Source: CAD feature listing. Evaluate the final solid. Frame: model axes, mm. Face numbers are marked on the shaded views. A direction names the side the tool comes from. Round coordinates to 2 decimals unless told otherwise and drop trailing zeros. Write each loop counter-clockwise with the first axis right and the second up, starting at its lowest first coordinate (ties: lowest second). Pieces come first, ordered by that corner, then holes. Notation, with made-up numbers: M 70,53.25 L 114,53.25 A32 cw 114,79.25 Z; hole C -18,21.25 d5. An arc over 180 degrees is marked long. Answer in a Markdown table with one row per item. Add a question column.
Item 1: Cut plane A-A on x = -10.5. Return loops of the section in (y, z).
Item 2: Cut plane C-C on y = -5.5. Return loops of the section in (x, z).
Item 3: Contact query for flat-ended pins moving along their axis: pin 1 (2 mm diameter, centred on x = -15.5, z = 7, fed in from -Y); pin 2 (3 mm diameter, centred on y = 19, z = 1.5, fed in from -X); pin 3 (5 mm diameter, centred on x = -2.5, z = 8, fed in from -Y). Output: stop coordinate, or through.
Item 4: Material intervals for probe 1 along Z at (x, y) = (-9.75, -3); probe 2 along X at (y, z) = (3, 9.75); probe 3 along Y at (x, z) = (-12.5, 6.25), sorted ascending.
Item 5: Set-up query: the marked faces 4, 5 and 6. Return all of +Z, -Z, +X, -X, +Y, -Y with unobstructed straight access to the full face (end or side cutting, diameter ignored); none if empty.
Item 6: Mould query, pull axis Z, two halves, no side actions, for the marked faces 1, 2 and 3. Classes: released by +Z, released by -Z, zero draft, split by the parting line, or undercut.
Item 7: Cut plane D-D on z = 5. Return loops of the section in (x, y).
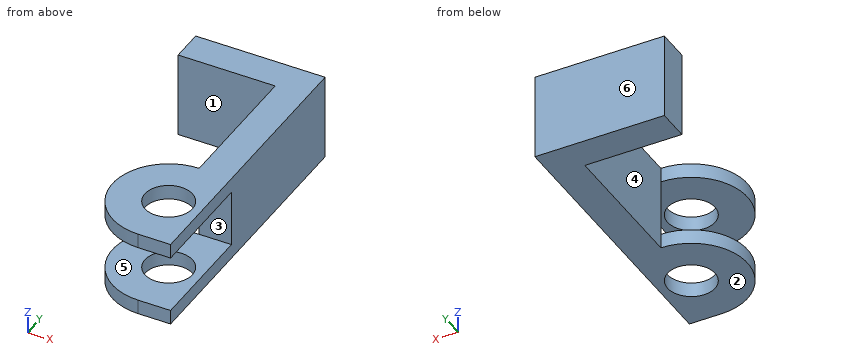
from build123d import *

# Parameters (mm, degrees)
SKETCH1_R           = 3.4925
BOSS_EXTRUDE1_DEPTH = 12.7
SKETCH2_W           = 25.4
SKETCH2_H           = 8.382
CUT_EXTRUDE1_DEPTH  = 16.51


with BuildPart() as part:
    # Sketch1 → Boss-Extrude1 (new body)
    with BuildSketch(Plane.XY):
        with BuildLine():
            Line((0, 0), (0, 25.4))
            Line((0, 25.4), (-19.05, 25.4))
            Line((-19.05, 25.4), (-19.05, 20.6375))
            Line((-19.05, 20.6375), (-4.7625, 20.6375))
            Line((-4.7625, 20.6375), (-4.7625, 0))
            ThreePointArc((-4.7625, 0), (-13.0175, -8.255), (-4.7625, -16.51))
            Line((-4.7625, -16.51), (0, -16.51))
            Line((0, -16.51), (0, 0))
        make_face()
        with Locations((-4.7625, -8.255)):
            Circle(SKETCH1_R, mode=Mode.SUBTRACT)
    extrude(amount=BOSS_EXTRUDE1_DEPTH)

    # Sketch2 → Cut-Extrude1 (cut)
    with BuildSketch(Plane.XZ.offset(16.51)):
        with Locations((-12.7, 6.35)):
            Rectangle(SKETCH2_W, SKETCH2_H)
    extrude(amount=-CUT_EXTRUDE1_DEPTH, mode=Mode.SUBTRACT)


solid = part.part
Results below:
| question | item | result |
|---|---|---|
| 1 | outline | M -14.19,0 L -2.32,0 L -2.32,2.16 L -14.19,2.16 Z; M -14.19,10.54 L -2.32,10.54 L -2.32,12.7 L -14.19,12.7 Z; M 20.64,0 L 25.4,0 L 25.4,12.7 L 20.64,12.7 Z |
| 2 | outline | M -12.54,0 L -6.91,0 L -6.91,2.16 L -12.54,2.16 Z; M -12.54,10.54 L -6.91,10.54 L -6.91,12.7 L -12.54,12.7 Z; M -2.62,0 L 0,0 L 0,2.16 L -2.62,2.16 Z; M -2.62,10.54 L 0,10.54 L 0,12.7 L -2.62,12.7 Z |
| 3 | pin 1 | y = 20.64 |
| 3 | pin 2 | x = -4.76 |
| 3 | pin 3 | y = 0 |
| 4 | probe 1 | 0 to 2.16, 10.54 to 12.7 |
| 4 | probe 2 | -4.76 to 0 |
| 4 | probe 3 | 20.64 to 25.4 |
| 5 | face 4 | +Z, -Z, -X |
| 5 | face 5 | +X, -X, -Y |
| 5 | face 6 | +Z, -Z, +X, -X, +Y |
| 6 | face 1 | zero draft |
| 6 | face 2 | released by -Z |
| 6 | face 3 | undercut |
| 7 | outline | M -19.05,20.64 L -4.76,20.64 L -4.76,0 L 0,0 L 0,25.4 L -19.05,25.4 Z |
